```python
from build123d import *

# Parameters (mm, degrees)
SKIZZE1_R                            = 3.5
AUFSATZ_LINEAR_AUSTRAGEN1_DEPTH      = 90
SKIZZE3_R                            = 1.4
AUFSATZ_LINEAR_AUSTRAGEN2_DEPTH      = 4.9
AUFSATZ_LINEAR_START                 = 4.9
SKIZZE4_R                            = 1.4
AUFSATZ_LINEAR_AUSTRAGEN3_DEPTH      = 4.9
SCHNITT_LINEAR_AUSTRAGEN7_DEPTH      = 96.028995575
SCHNITT_LINEAR_AUSTRAGEN7_DEPTH_BACK = 96.028995575
SKIZZE11_W                           = 4.192865468
SKIZZE11_H                           = 8.003816725
SCHNITT_LINEAR_AUSTRAGEN8_DEPTH      = 96.028995575
SCHNITT_LINEAR_AUSTRAGEN8_DEPTH_BACK = 96.028995575
SKIZZE12_W                           = 3.359837997
SKIZZE12_H                           = 7.994786778


with BuildPart() as part:
    # Skizze1 → Aufsatz-Linear austragen1 (new body)
    with BuildSketch(Plane.XY):
        with Locations(Location((0, 0, 0), (0, 0, 180))):
            Circle(SKIZZE1_R)
    extrude(amount=AUFSATZ_LINEAR_AUSTRAGEN1_DEPTH)

    # Skizze3 → Aufsatz-Linear austragen2 (add)
    with BuildSketch(Plane.XY.offset(90)):
        Circle(SKIZZE3_R)
    extrude(amount=AUFSATZ_LINEAR_AUSTRAGEN2_DEPTH)

    # Skizze4 → Aufsatz-Linear austragen3 (add)
    with BuildSketch(Plane(origin=(0, 0, 0), x_dir=(-1, 0, 0), z_dir=(0, 0, -1)).offset(AUFSATZ_LINEAR_START)):
        with Locations(Location((0, 0, 0), (0, 0, 180))):
            Circle(SKIZZE4_R)
    extrude(amount=-AUFSATZ_LINEAR_AUSTRAGEN3_DEPTH)

    # Skizze11 → Schnitt-Linear austragen7 (cut, two sides: drawn at the far end of the back side and taken through both)
    with BuildSketch(Plane.XY.offset(90).offset(-SCHNITT_LINEAR_AUSTRAGEN7_DEPTH_BACK)):
        with Locations((3.096432734, -0.133552217)):
            Rectangle(SKIZZE11_W, SKIZZE11_H)
    extrude(amount=SCHNITT_LINEAR_AUSTRAGEN7_DEPTH + SCHNITT_LINEAR_AUSTRAGEN7_DEPTH_BACK, mode=Mode.SUBTRACT)

    # Skizze12 → Schnitt-Linear austragen8 (cut, two sides: drawn at the far end of the back side and taken through both)
    with BuildSketch(Plane.XY.offset(90).offset(-SCHNITT_LINEAR_AUSTRAGEN8_DEPTH_BACK)):
        with Locations((-2.679918999, -0.138067191)):
            Rectangle(SKIZZE12_W, SKIZZE12_H)
    extrude(amount=SCHNITT_LINEAR_AUSTRAGEN8_DEPTH + SCHNITT_LINEAR_AUSTRAGEN8_DEPTH_BACK, mode=Mode.SUBTRACT)


solid = part.part
```
Design review of the part built by this model. Coordinates are the model's own, in mm. A direction names the side the tool comes from. Coordinates: 2 decimals unless noted, no trailing zeros. Loops run counter-clockwise (first coordinate to the right, second up) from the corner with the lowest first, then second, coordinate; pieces in that order, holes last. Notation, with made-up numbers: (1, -35) -> (25, -35) arc R5 ccw to (25, -27) -> close; hole circle Ø9 at (31, 21). An arc over 180 degrees is marked (long way). Answer as a JSON object with one key per item and string values.
Q1. To check wall thickness, follow L1, parallel to Z at x = 0.35, y = 3; L2, parallel to Y at x = -0.1, z = 21.5; L3, parallel to Y at x = 0.85, z = 76. State the ranges of each line that lie inside material, in increasing order.
Answer block:
{"L1": "z = 0 to 90", "L2": "y = -3.5 to 3.5", "L3": "y = -3.4 to 3.4"}
Q2. Tool access review of faces 1 (the cylindrical face through (0, -1.4, -2.5)), 2 (the cylindrical face through (0, 1.4, 92.4)), 3 (the cylindrical face through (0, 1.4, -2.5)): name each direction out of +Z, -Z, +X, -X, +Y, -Y from which nothing blocks a thin tool from reaching the whole face with its end or side.
Answer block:
{"face 1": "-Z, -Y", "face 2": "+Z, +Y", "face 3": "-Z, +Y"}
Q3. Take a section at B-B on y = -2.25. Give the boundary of the cut face in (x, z).
Answer block:
{"outline": "(-1, 0) -> (1, 0) -> (1, 90) -> (-1, 90) -> close"}
Q4. Take a section at A-A on x = 0. Give the boundary of the cut face in (y, z).
Answer block:
{"outline": "(-3.5, 0) -> (-1.4, 0) -> (-1.4, -4.9) -> (1.4, -4.9) -> (1.4, 0) -> (3.5, 0) -> (3.5, 90) -> (1.4, 90) -> (1.4, 94.9) -> (-1.4, 94.9) -> (-1.4, 90) -> (-3.5, 90) -> close"}
Q5. Clearance check with a flat-ended pin moving along its axis: pin 1 Ø0.6 at (x, y) = (-0.5, 2.5) entering from -Z. State where the tip first meets the part, or that it passes through.
Answer block:
{"pin 1": "stops at z = 0"}
